Could you check a few things on this drawing? It's one solid part, dimensions in mm from its lowest x, y, z. A direction names the side the tool comes from. Coordinates: 2 decimals unless noted, no trailing zeros. Order: outer loops, then holes, each group sorted by start corner. A loop starts at its lowest first (then second) coordinate and runs counter-clockwise, first axis right, second up. Notation, with made-up numbers: (-31, 50.5) -> (4, 50.5) arc R32 ccw to (4, 87.5) -> close; hole circle Ø2 at (0.5, -30). An arc over 180 degrees is marked (long way). Use a Markdown table: item, result. Add a question column.
1. Suppose I cut it at B-B, the plane x = 63.5. List the corners of the cut face in (y, z) for me.
2. For the marked faces 1, 2 and 3, which set-ups out of +Z, -Z, +X, -X, +Y, -Y let a thin tool reach every point of the face, with its end or its side?
3. If I drill on line 1 along Z through (x, y) = (62, 319.5); line 2 along Y through (x, z) = (22, 66.5); line 3 along X through (y, z) = (175, 64.5), over which ranges is the centre line in solid material (lowest first)? Write a range as from..to.
4. Suppose I cut it at A-A, the plane z = 63.5. List the corners of the cut face in (x, y) for me, then the cut area to 3 significant figures.
5. For pin 1 Ø10 at (x, y) = (102.5, 291.5) entering from -Z; pin 2 Ø5 at (y, z) = (198.5, 93) entering from +X; pin 3 Ø1 at (y, z) = (248.5, 32) entering from +X, each with a flat end and sliding along its axis, tell me the tip position at first contact or that it passes through.
6. Suppose I cut it at C-C, the plane y = 249.5. List the corners of the cut face in (x, z) for me.
7. Suppose I cut it at D-D, the plane x = 119.5. List the corners of the cut face in (y, z) for me.
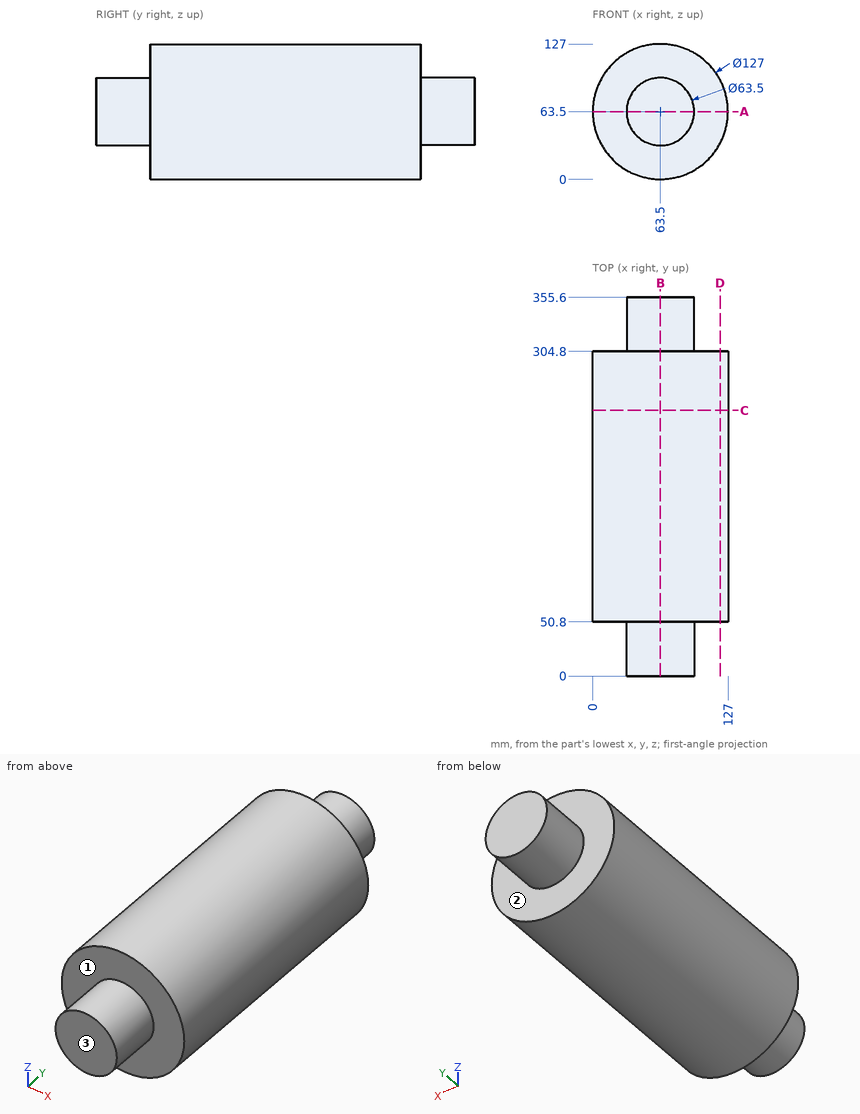
Worked out:
| question | item | result |
|---|---|---|
| 1 | outline | (0, 31.75) -> (50.8, 31.75) -> (50.8, 0) -> (304.8, 0) -> (304.8, 31.75) -> (355.6, 31.75) -> (355.6, 95.25) -> (304.8, 95.25) -> (304.8, 127) -> (50.8, 127) -> (50.8, 95.25) -> (0, 95.25) -> close |
| 2 | face 1 | -Y |
| 2 | face 2 | +Y |
| 2 | face 3 | +Z, -Z, +X, -X, -Y |
| 3 | line 1 | z = 31.79..95.21 |
| 3 | line 2 | y = 50.8..304.8 |
| 3 | line 3 | x = 0.01..126.99 |
| 4 | outline | (0, 50.8) -> (31.75, 50.8) -> (31.75, 0) -> (95.25, 0) -> (95.25, 50.8) -> (127, 50.8) -> (127, 304.8) -> (95.25, 304.8) -> (95.25, 355.6) -> (31.75, 355.6) -> (31.75, 304.8) -> (0, 304.8) -> close |
| 4 | area | 38,700 mm² |
| 5 | pin 1 | stops at z = 9.87 |
| 5 | pin 2 | stops at x = 120.97 |
| 5 | pin 3 | stops at x = 118.92 |
| 6 | outline | circle Ø127 at (63.5, 63.5) |
| 7 | outline | (50.8, 33.56) -> (304.8, 33.56) -> (304.8, 93.44) -> (50.8, 93.44) -> close |
